For this review, use the dimensioned drawing (mm, ordinates from the lowest corner) and the shaded views. A direction names the side the tool comes from. Coordinates: 2 decimals unless noted, no trailing zeros. Loops run counter-clockwise (first coordinate to the right, second up) from the corner with the lowest first, then second, coordinate; pieces in that order, holes last. Notation, with made-up numbers: (-19.5, -21.75) - (29.5, -21.75) arc R8 ccw to (29.5, -11.75) - close; hole circle Ø2 at (-40, -31). An arc over 180 degrees is marked (long way). Answer in a Markdown table with one row per item. Add a question column.
(1) We need section C-C, the plane y = 21. Write out the cut boundary in (x, z), plus the area to 3 significant figures.
(2) For the marked faces 4 and 5, list the 3-axis set-ups (+Z, -Z, +X, -X, +Y, -Y) from which the entire face can be reached by the end or side of a thin tool; tool diameter is ignored.
(3) We need section A-A, the plane x = 27.5. Write out the cut boundary in (y, z), plus the area to 3 significant figures.
(4) Clearance check with flat-ended pins moving along their axes: pin 1 (1.5 mm diameter, centred on y = 3, z = 5.5, fed in from +X); pin 2 (4 mm diameter, centred on y = 27, z = 2, fed in from +X). State where each tip first meets the part, or that it passes through.
(5) To check wall thickness, follow L1, parallel to Y at x = 27.5, z = 7; L2, parallel to X at y = 5.5, z = 7; L3, parallel to Y at x = 29.5, z = 5. State the ranges of each line that lie inside material, in increasing order. Write a range as [from, to].
(6) We need section B-B, the plane z = 1.75. Write out the cut boundary in (x, y), plus the area to 3 significant figures.
(7) The part is to be moulded in two halves that separate along Y. For the marked faces 1, 2 and 3, say which applies: released by +Y, released by -Y, zero draft, split by the parting line, or undercut.
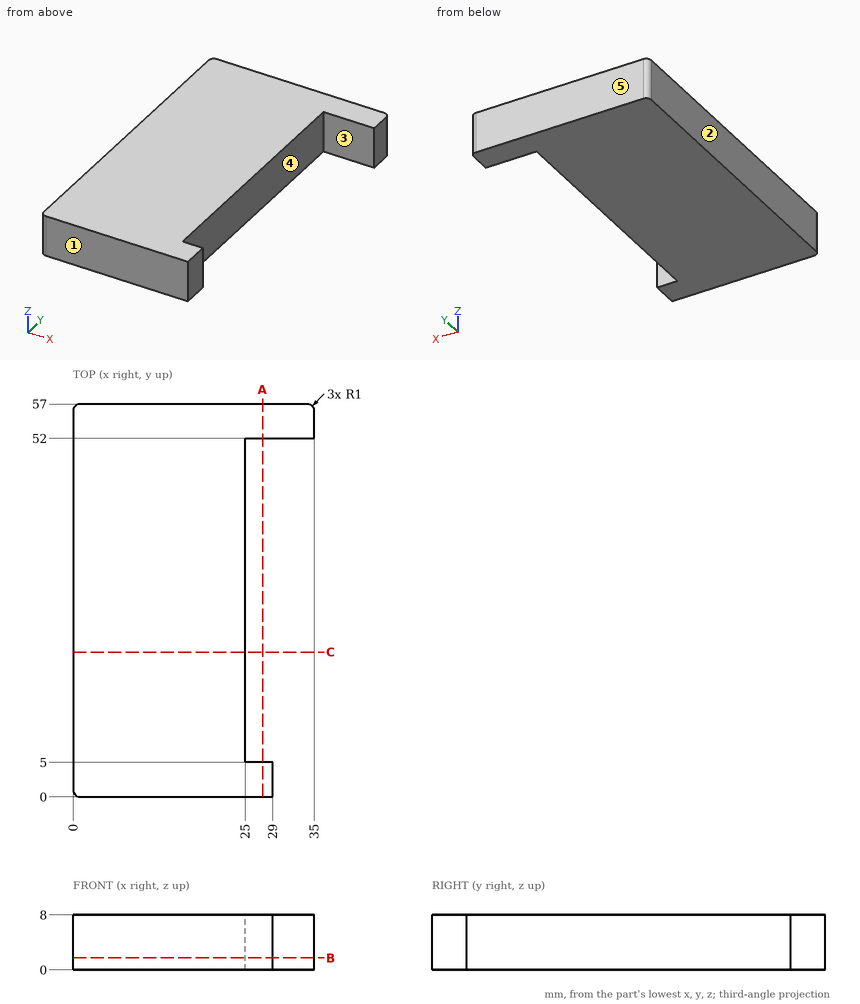
Responses:
| question | item | result |
|---|---|---|
| 1 | outline | (0, 0) - (25, 0) - (25, 8) - (0, 8) - close |
| 1 | area | 200 mm2 |
| 2 | face 4 | +Z, -Z, +X |
| 2 | face 5 | +Z, -Z, +X, -X, +Y |
| 3 | outline | (0, 0) - (5, 0) - (5, 8) - (0, 8) - close; (52, 0) - (57, 0) - (57, 8) - (52, 8) - close |
| 3 | area | 80.0 mm2 |
| 4 | pin 1 | stops at x = 29 |
| 4 | pin 2 | stops at x = 25 |
| 5 | L1 | y = [0, 5], [52, 57] |
| 5 | L2 | x = [0, 25] |
| 5 | L3 | y = [52, 57] |
| 6 | outline | (0, 1) arc R1 ccw to (1, 0) - (29, 0) - (29, 5) - (25, 5) - (25, 52) - (35, 52) - (35, 56) arc R1 ccw to (34, 57) - (1, 57) arc R1 ccw to (0, 56) - close |
| 6 | area | 1,490 mm2 |
| 7 | face 1 | released by -Y |
| 7 | face 2 | zero draft |
| 7 | face 3 | undercut |
